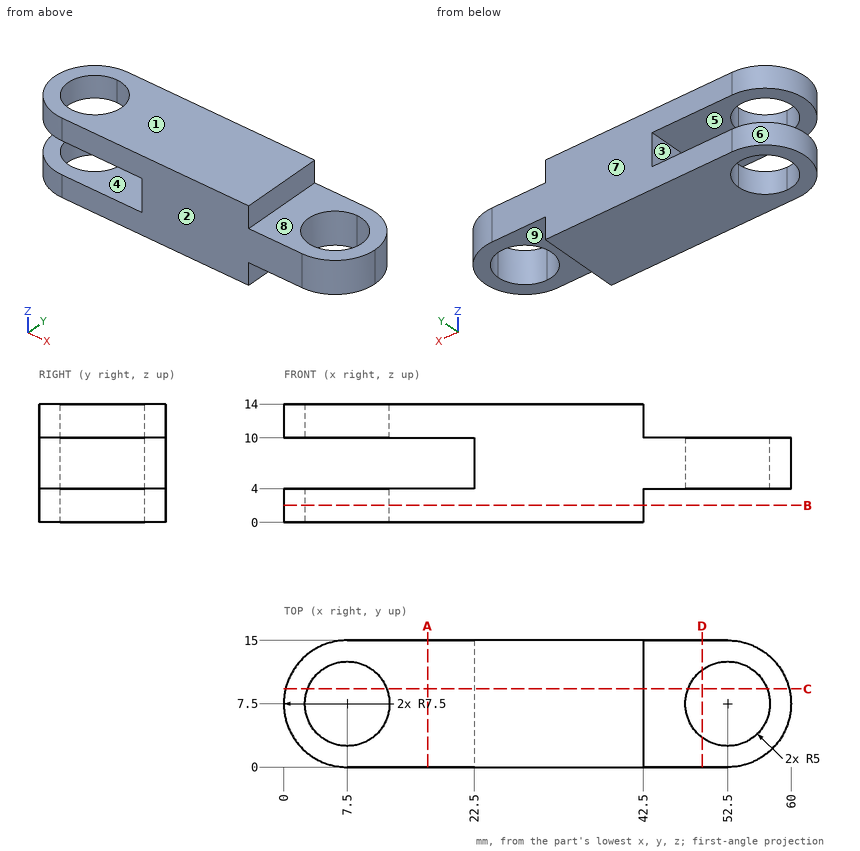
Answer from the drawing. Dimensions are ordinates in mm from the lowest x, y and z of the part. A direction names the side the tool comes from. Round coordinates to 2 decimals unless told otherwise and drop trailing zeros. Write each loop counter-clockwise with the first axis right and the second up, starting at its lowest first coordinate (ties: lowest second). Pieces come first, ordered by that corner, then holes. Notation, with made-up numbers: (26, 31) -> (44, 31) arc R22 ccw to (44, 46) -> close; hole circle Ø11 at (53, 69.25). An arc over 180 degrees is marked (long way). Answer in a Markdown table with one row per item. Add a question column.
1) Which of the six approach directions +Z, -Z, +X, -X, +Y, -Y give full straight-line access (tool end or side, diameter ignored) to the marked faces 5, 6, 7, 8 and 9?
2) Find section A-A, the plane x = 17. Determine the outline of the cut face in (y, z).
3) Determine the mould class of the marked faces 1, 2, 3 and 4 for opening direction Z: pulls with the +Z half, pulls with the -Z half, needs draft (parallel to the pull), parting line crosses it, or undercut.
4) Consider line 1 (Z direction, x = 14, y = 8.5); line 2 (X direction, y = 11, z = 1.25); line 3 (Z direction, x = 58.5, y = 9). Determine where each line is inside the solid, lowest interval first.
5) Find section D-D, the plane x = 49.5. Determine the outline of the cut face in (y, z).
6) Given P1, Ø1.8, axis at y = 8.5, z = 7, coming from the -X side; P2, Ø1.5, axis at x = 29.5, y = 8, coming from the -Z side; P3, Ø2, axis at y = 10, z = 9, coming from the +X side; P4, Ø4.5, axis at x = 48.5, y = 10.5, coming from the -Z side, each flat-ended and moving along its own axis, determine where each tip first touches the part or whether it passes through.
7) Find section B-B, the plane z = 2. Determine the outline of the cut face in (x, y).
8) Find section C-C, the plane y = 9.25. Determine the outline of the cut face in (x, z).
Findings below:
| question | item | result |
|---|---|---|
| 1 | face 5 | -X, +Y, -Y |
| 1 | face 6 | +Z, -Z, -X |
| 1 | face 7 | +Z, -Z, +X, -X, +Y |
| 1 | face 8 | +Z, +X, +Y, -Y |
| 1 | face 9 | -Z, +X, +Y, -Y |
| 2 | outline | (0, 0) -> (15, 0) -> (15, 4) -> (0, 4) -> close; (0, 10) -> (15, 10) -> (15, 14) -> (0, 14) -> close |
| 3 | face 1 | pulls with the +Z half |
| 3 | face 2 | needs draft |
| 3 | face 3 | undercut |
| 3 | face 4 | undercut |
| 4 | line 1 | 0 to 4, 10 to 14 |
| 4 | line 2 | 0.87 to 3.93, 11.07 to 42.5 |
| 4 | line 3 | 4 to 10 |
| 5 | outline | (0, 4) -> (3.5, 4) -> (3.5, 10) -> (0, 10) -> close; (11.5, 4) -> (15, 4) -> (15, 10) -> (11.5, 10) -> close |
| 6 | P1 | x = 22.5 |
| 6 | P2 | z = 0 |
| 6 | P3 | x = 59.85 |
| 6 | P4 | z = 4 |
| 7 | outline | (7.5, 0) -> (42.5, 0) -> (42.5, 15) -> (7.5, 15) arc R7.5 ccw to start; hole circle Ø10 at (7.5, 7.5) |
| 8 | outline | (0.21, 0) -> (2.82, 0) -> (2.82, 4) -> (0.21, 4) -> close; (0.21, 10) -> (2.82, 10) -> (2.82, 14) -> (0.21, 14) -> close; (12.18, 0) -> (42.5, 0) -> (42.5, 4) -> (47.82, 4) -> (47.82, 10) -> (42.5, 10) -> (42.5, 14) -> (12.18, 14) -> (12.18, 10) -> (22.5, 10) -> (22.5, 4) -> (12.18, 4) -> close; (57.18, 4) -> (59.79, 4) -> (59.79, 10) -> (57.18, 10) -> close |
